Here's how the part is built. I have some questions about the finished solid (model axes, mm). Round coordinates to 2 decimals unless told otherwise and drop trailing zeros. Loops run counter-clockwise (first coordinate to the right, second up) from the corner with the lowest first, then second, coordinate; pieces in that order, holes last. Notation, with made-up numbers: M 80.25,55 L 97.25,55 A9 ccw 97.25,61 Z; hole C 30.5,68 d1. An arc over 180 degrees is marked long. Answer as a JSON object with one key per item and string values.
from build123d import *

# Parameters (mm, degrees)
F0_W     = 1
F0_H     = 10
F2_R     = 1.5
F3_DEPTH = 10


# Not quite as in the source:
# - a pattern or mirror of a feature is missing from the dataset's text; its kind, count and spacing are read off the source's solid


with BuildPart() as f1:
    # F0 (on Front) → F1 (revolve)
    with BuildSketch(Plane.XZ):
        with Locations((55.5, 5)):
            Rectangle(F0_W, F0_H)
    revolve(axis=Axis((0, 0, 25.0742025673), (0, 0, 1)))

    # F2 (on Top) → F3 (join)
    with BuildSketch(Plane.XY):
        with BuildLine():
            ThreePointArc((55.8974828375, -3.3869473613), (56.2759455722, -2.6625949972), (57.0683229814, -2.4624489744))
            ThreePointArc((57.0683229814, -2.4624489744), (60, 0), (57.0683229814, 2.4624489744))
            ThreePointArc((57.0683229814, 2.4624489744), (56.2759455722, 2.6625949972), (55.8974828375, 3.3869473613))
            Line((55.8974828375, 3.3869473613), (55.3983981693, 3.3567067599))
            ThreePointArc((55.3983981693, 3.3567067599), (55.5, 0), (55.3983981693, -3.3567067599))
            Line((55.3983981693, -3.3567067599), (55.8974828375, -3.3869473613))
        make_face()
        with Locations((57.5, 0)):
            Circle(F2_R, mode=Mode.SUBTRACT)
    f3 = extrude(amount=F3_DEPTH)

    # F3_copies: F3 across plane
    add(f3.mirror(Plane(origin=(0, 0, 0), x_dir=(0, 0, -1), z_dir=(-1, 0, 0))))


solid = f1.part
Item 1: I'm going to push flat-ended pins straight in: pin 1 Ø1 at (x, z) = (-37, 5.5) entering from -Y; pin 2 Ø2 at (y, z) = (2.5, 4) entering from +X; pin 3 Ø5 at (y, z) = (5.5, 6) entering from +X. Where does each tip first touch, or does it pass through?
Resolved:
{"pin 1": "y = -42.47", "pin 2": "x = 59.5", "pin 3": "x = 56"}
Item 2: Please list where these lines run through material, in increasing order: probe 1 along Y at (x, z) = (57.5, 4.75); probe 2 along Y at (x, z) = (47, 3.25); probe 3 along X at (y, z) = (35.5, 5.75). Write a range as from..to.
Resolved:
{"probe 1": "-2.5..-1.5, 1.5..2.5", "probe 2": "-30.45..-28.57, 28.57..30.45", "probe 3": "-43.31..-42.01, 42.01..43.31"}
Item 3: If we mould it in two halves opening along X, with no side actions, what happens to faces 1 (the face through (59, 0, 5)), 2 (the face through (36, 42, 0)), 3 (the face through (-1.184, -55.987, 5.07))? For each: pulls with the +X half, pulls with the -X half, needs draft (parallel to the pull), parting line crosses it, or undercut.
Resolved:
{"face 1": "undercut", "face 2": "needs draft", "face 3": "parting line crosses it"}
Item 4: I want a section at B-B, the plane x = 0. Please give me the cut outline in (y, z).
Resolved:
{"outline": "M -56,0 L -55,0 L -55,10 L -56,10 Z; M 55,0 L 56,0 L 56,10 L 55,10 Z"}
Item 5: I want a section at A-A, the plane y = 0. Please give me the cut outline in (x, z).
Resolved:
{"outline": "M -60,0 L -59,0 L -59,10 L -60,10 Z; M -56,0 L -55,0 L -55,10 L -56,10 Z; M 55,0 L 56,0 L 56,10 L 55,10 Z; M 59,0 L 60,0 L 60,10 L 59,10 Z"}
Item 6: I want a section at C-C, the plane y = -44. Please give me the cut outline in (x, z).
Resolved:
{"outline": "M -34.64,0 L -33,0 L -33,10 L -34.64,10 Z; M 33,0 L 34.64,0 L 34.64,10 L 33,10 Z"}
